```python
from build123d import *

# Parameters (mm, degrees)
F1_DEPTH = 6.35


with BuildPart() as f1:
    # F0 (on Front) → F1 (new body, symmetric)
    with BuildSketch(Plane.XZ):
        with BuildLine():
            Line((-38.1, -25.4), (38.1, -25.4))
            ThreePointArc((38.1, -25.4), (47.0802561211, -21.6802561211), (50.8, -12.7))
            Line((50.8, -12.7), (50.8, 12.7))
            ThreePointArc((50.8, 12.7), (47.0802561211, 21.6802561211), (38.1, 25.4))
            Line((38.1, 25.4), (25.4, 25.4))
            Line((25.4, 25.4), (25.4, 0))
            Line((25.4, 0), (-25.4, 0))
            Line((-25.4, 0), (-25.4, 25.4))
            Line((-25.4, 25.4), (-38.1, 25.4))
            ThreePointArc((-38.1, 25.4), (-47.0802561211, 21.6802561211), (-50.8, 12.7))
            Line((-50.8, 12.7), (-50.8, -12.7))
            ThreePointArc((-50.8, -12.7), (-47.0802561211, -21.6802561211), (-38.1, -25.4))
        make_face()
    extrude(amount=F1_DEPTH, both=True)


solid = f1.part
```
Here's how the part is built. I have some questions about the finished solid (model axes, mm). A direction names the side the tool comes from. Give positions to 0.01 mm unless a question says otherwise; leave off trailing zeros. Order: outer loops, then holes, each group sorted by start corner. A loop starts at its lowest first (then second) coordinate and runs counter-clockwise, first axis right, second up. Notation, with made-up numbers: M 64.5,17.5 L 119.5,17.5 A24 cw 119.5,37.5 Z; hole C -6,88.5 d1. An arc over 180 degrees is marked long. Use a Markdown table: item, result. Add a question column.
1. Suppose I cut it at D-D (x = 8). List the corners of the cut face in (y, z) for me.
2. If we mould it in two halves opening along X, with no side actions, what happens to faces 3 (the cylindrical face through (-47.18, -0.09, -21.58)), 4 (the flat face through (-25.4, 0, 13)), 5 (the flat face through (25.4, 0, 13)), 6 (the flat face through (-32, 0, 25.4))? For each: +X half, -X half, draft (parallel to the pull), parting line (faces both ways), or undercut.
3. For pin 1 Ø6.5 at (x, y) = (-2, 2.5) entering from +Z; pin 2 Ø4 at (y, z) = (-2, 15) entering from -X, each with a flat end and sliding along its axis, tell me the tip position at first contact or that it passes through.
4. Suppose I cut it at A-A (z = 6.5). List the corners of the cut face in (x, y) for me.
5. I need wall thicknesses on probe 1 along X at (y, z) = (-3, 9); probe 2 along Z at (x, y) = (25, -1.75); probe 3 along X at (y, z) = (0.75, 20.5). Which ranges of each line are inside material? Lowest first, please. Write a range as from..to.
6. Suppose I cut it at B-B (y = -0.75). List the corners of the cut face in (x, z) for me.
7. Suppose I cut it at C-C (z = 18). List the corners of the cut face in (x, y) for me, and give its area (3 significant figures).
8. On a 3-axis mill with a long thin cutter (end or side, diameter ignored), from which of +Z, -Z, +X, -X, +Y, -Y can I reach the whole of each face in a straight line? I mean faces 1 (the flat face through (0, 0, 0)), 2 (the cylindrical face through (46.98, -0.09, -21.78)). Say none if no direction works.
Results list:
| question | item | result |
|---|---|---|
| 1 | outline | M -6.35,-25.4 L 6.35,-25.4 L 6.35,0 L -6.35,0 Z |
| 2 | face 3 | -X half |
| 2 | face 4 | undercut |
| 2 | face 5 | undercut |
| 2 | face 6 | draft |
| 3 | pin 1 | stops at z = 0 |
| 3 | pin 2 | stops at x = -50.8 |
| 4 | outline | M -50.8,-6.35 L -25.4,-6.35 L -25.4,6.35 L -50.8,6.35 Z; M 25.4,-6.35 L 50.8,-6.35 L 50.8,6.35 L 25.4,6.35 Z |
| 5 | probe 1 | x = -50.8..-25.4, 25.4..50.8 |
| 5 | probe 2 | z = -25.4..0 |
| 5 | probe 3 | x = -48.12..-25.4, 25.4..48.12 |
| 6 | outline | M -50.8,-12.7 A12.7 ccw -38.1,-25.4 L 38.1,-25.4 A12.7 ccw 50.8,-12.7 L 50.8,12.7 A12.7 ccw 38.1,25.4 L 25.4,25.4 L 25.4,0 L -25.4,0 L -25.4,25.4 L -38.1,25.4 A12.7 ccw -50.8,12.7 Z |
| 7 | outline | M -49.64,-6.35 L -25.4,-6.35 L -25.4,6.35 L -49.64,6.35 Z; M 25.4,-6.35 L 49.64,-6.35 L 49.64,6.35 L 25.4,6.35 Z |
| 7 | area | 616 mm² |
| 8 | face 1 | +Z, +Y, -Y |
| 8 | face 2 | -Z, +X, +Y, -Y |
